Can you work these out from the drawing? Everything is in mm from the part's minimum corner. A direction names the side the tool comes from. Give positions to 0.01 mm unless a question says otherwise; leave off trailing zeros. Loops run counter-clockwise (first coordinate to the right, second up) from the corner with the lowest first, then second, coordinate; pieces in that order, holes last. Notation, with made-up numbers: (36.25, 10.5) -> (52.25, 10.5) arc R23 cw to (52.25, 41.5) -> close; hole circle Ø3 at (49, 30.25). An arc over 180 degrees is marked (long way). Write item = value, one per line. Start each with the question number.
1) I want a section at C-C (x = 4.5). List the corners of the cut face in (y, z) for me.
2) I want a section at D-D (y = 3.25). List the corners of the cut face in (x, z) for me, and give its area (3 significant figures).
3) On a 3-axis mill with a long thin cutter (end or side, diameter ignored), from which of +Z, -Z, +X, -X, +Y, -Y can I reach the whole of each face in a straight line? I mean the marked faces 5 and 6. Say none if no direction works.
4) I'm going to push flat-ended pins straight in: pin 1 Ø5 at (x, z) = (13, 7) entering from +Y; pin 2 Ø1 at (x, z) = (2, 5) entering from -Y; pin 3 Ø1 at (y, z) = (11, 2.5) entering from +X. Where does each tip first touch, or does it pass through?
5) I want a section at B-B (y = 8). List the corners of the cut face in (x, z) for me, and give its area (3 significant figures).
6) I need wall thicknesses on probe 1 along Y at (x, z) = (8, 4); probe 2 along Z at (x, y) = (15.25, 5.25); probe 3 along Y at (x, z) = (10.25, 7). Which ranges of each line are inside material? Lowest first, please. Write a range as from..to.
7) If we mould it in two halves opening along Z, with no side actions, what happens to the marked faces 1, 2, 3 and 4? For each: +Z half, -Z half, draft (parallel to the pull), parting line (faces both ways), or undercut.
8) I want a section at A-A (x = 14.75). List the corners of the cut face in (y, z) for me, and give its area (3 significant figures).
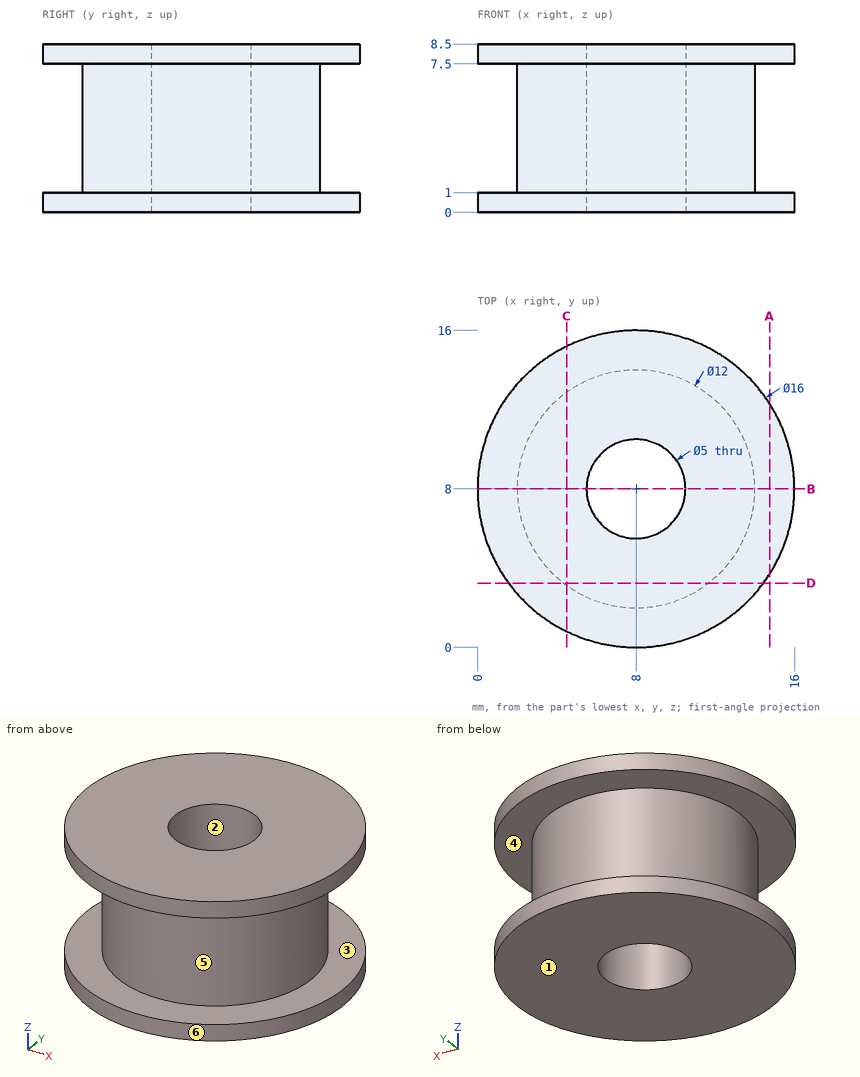
Answer list:
q1.outline = (0.81, 0) -> (15.19, 0) -> (15.19, 1) -> (12.87, 1) -> (12.87, 7.5) -> (15.19, 7.5) -> (15.19, 8.5) -> (0.81, 8.5) -> (0.81, 7.5) -> (3.13, 7.5) -> (3.13, 1) -> (0.81, 1) -> close
q2.outline = (1.56, 0) -> (14.44, 0) -> (14.44, 1) -> (11.67, 1) -> (11.67, 7.5) -> (14.44, 7.5) -> (14.44, 8.5) -> (1.56, 8.5) -> (1.56, 7.5) -> (4.33, 7.5) -> (4.33, 1) -> (1.56, 1) -> close
q2.area = 73.4 mm^2
q3.face_5 = none
q3.face_6 = +Z, -Z
q4.pin_1 = 15.58
q4.pin_2 = 5.6
q4.pin_3 = 13.45
q5.outline = (0, 0) -> (5.5, 0) -> (5.5, 8.5) -> (0, 8.5) -> (0, 7.5) -> (2, 7.5) -> (2, 1) -> (0, 1) -> close; (10.5, 0) -> (16, 0) -> (16, 1) -> (14, 1) -> (14, 7.5) -> (16, 7.5) -> (16, 8.5) -> (10.5, 8.5) -> close
q5.area = 67.5 mm^2
q6.probe_1 = 2..5.5, 10.5..14
q6.probe_2 = 0..1, 7.5..8.5
q6.probe_3 = 2.44..6.91, 9.09..13.56
q7.face_1 = -Z half
q7.face_2 = draft
q7.face_3 = undercut
q7.face_4 = undercut
q8.outline = (3.71, 0) -> (12.29, 0) -> (12.29, 1) -> (3.71, 1) -> close; (3.71, 7.5) -> (12.29, 7.5) -> (12.29, 8.5) -> (3.71, 8.5) -> close
q8.area = 17.2 mm^2
